from build123d import *

# Parameters (mm, degrees)
F0_W          = 20
F0_H          = 40
F0_R          = 1.75
F1_DEPTH      = 14
F2_W          = 20
F2_H          = 8.7217967697
F2_H_2        = 9.1349255253
F3_DEPTH      = 10
F4_R          = 6
F5_DEPTH      = 14
F5_DEPTH_BACK = 20


with BuildPart() as f1:
    # F0 (on Top) → F1 (new body)
    with BuildSketch(Plane.XY):
        Rectangle(F0_W, F0_H)
        with Locations((0, -15)):
            Circle(F0_R, mode=Mode.SUBTRACT)
        with Locations((0, 15)):
            Circle(F0_R, mode=Mode.SUBTRACT)
    extrude(amount=F1_DEPTH)

    # F2 (on face) → F3 (cut)
    with BuildSketch(Plane.XY.offset(14)):
        Polygon((-6.0882685902, -5.1451905284), (-3.75, -6.4951905284), (-1.3077413577, -7.8650744747), (6.4248711306, 5.5282032303), (1.6617314098, 8.2782032303), align=None)
        with Locations((0, 15.6391016151)):
            Rectangle(F2_W, F2_H)
        with Locations((0, -15.4325372373)):
            Rectangle(F2_W, F2_H_2)
    extrude(amount=-F3_DEPTH, mode=Mode.SUBTRACT)

    # F4 (on face) → F5 (cut, two sides)
    with BuildSketch(Plane(origin=(-2.3382685902, 1.35, 0), x_dir=(0.5, 0.8660254038, 0), z_dir=(0.8660254038, -0.5, 0))) as f5_sk:
        with Locations((0.25, 12.454691343)):
            Circle(F4_R)
    extrude(amount=-F5_DEPTH, mode=Mode.SUBTRACT)
    extrude(f5_sk.sketch, amount=F5_DEPTH_BACK, mode=Mode.SUBTRACT)


solid = f1.part
Geometry: final body of the model. Coordinates: model frame, mm. A direction names the side the tool comes from. Round coordinates to 2 decimals unless told otherwise and drop trailing zeros. Loops run counter-clockwise (first coordinate to the right, second up) from the corner with the lowest first, then second, coordinate; pieces in that order, holes last. Notation, with made-up numbers: (50, 11.25) - (66, 11.25) arc R28 cw to (66, 40.25) - close; hole circle Ø7 at (20, 51.5). An arc over 180 degrees is marked (long way). Write each question's results on one line, items separated by ' | '. Start each with the question number.
1) Cut plane C-C on z = 11. Return loops of the section in (x, y), then the cut area to 3 significant figures.
2) Cut plane B-B on y = 15. Return loops of the section in (x, z).
3) Cut plane D-D on z = 2.25. Return loops of the section in (x, y), then the cut area to 3 significant figures.
4) Cut plane A-A on z = 4.5. Return loops of the section in (x, y), then the cut area to 3 significant figures.
5) Mould query, pull axis Y, two halves, no side actions, for faces 4 (the face through (0, 20, 2)), 5 (the face through (-10, 0, 5)), 6 (the face through (2.504, -1.262, 5.737)), 7 (the face through (0, -10.865, 9)). Classes: released by +Y, released by -Y, zero draft, split by the parting line, or undercut.
6) Line query: probe 1 along Y at (x, z) = (0, 0.9); probe 2 along X at (y, z) = (15, 2); probe 3 along Z at (x, y) = (1, 4). Output: solid intervals per line, ascending. Write a range as [from, to].
7) Access query for faces 1 (the face through (0, -17, 4)), 2 (the face through (0, 18, 4)), 3 (the face through (0, 0, 4)). Directions: +Z, -Z, +X, -X, +Y, -Y. A direction counts if a zero-diameter tool reaches every point of the face in a straight line with its end or side. Return the directions, or none.
8) First-contact query: P1, Ø3, axis at x = 0, y = 15, coming from the -Z side; P2, Ø4, axis at x = 7, y = -7.5, coming from the +Z side; P3, Ø5, axis at x = 6.5, y = -6, coming from the -Z side; P4, Ø1, axis at y = 6.5, z = 12.5, coming from the -X side. Flat tips, straight axial feed; report the tip coordinate or a pass-through.
Verdict:
1) outline: (-10, -10.87) - (7.68, -10.87) - (-0.36, -6.22) - (-1.31, -7.87) - (-3.75, -6.5) - (-6.09, -5.15) - (-5.12, -3.47) - (-10, -0.66) - close; (-7.39, 11.28) - (0.7, 6.61) - (1.66, 8.28) - (6.42, 5.53) - (5.46, 3.86) - (10, 1.24) - (10, 11.28) - close | area: 156 mm2
2) outline: (-10, 0) - (-1.75, 0) - (-1.75, 4) - (-10, 4) - close; (1.75, 0) - (10, 0) - (10, 4) - (1.75, 4) - close
3) outline: (-10, -20) - (10, -20) - (10, 20) - (-10, 20) - close; hole circle Ø3.5 at (0, -15); hole circle Ø3.5 at (0, 15) | area: 781 mm2
4) outline: (-10, -10.87) - (10, -10.87) - (10, 11.28) - (-10, 11.28) - close; hole (-6.09, -5.15) - (-3.75, -6.5) - (-1.31, -7.87) - (6.42, 5.53) - (1.66, 8.28) - close | area: 358 mm2
5) face 4: released by +Y | face 5: zero draft | face 6: undercut | face 7: released by -Y
6) probe 1: y = [-20, -16.75], [-13.25, 13.25], [16.75, 20] | probe 2: x = [-10, -1.75], [1.75, 10] | probe 3: z = [0, 4]
7) face 1: +Z, +X, -X, -Y | face 2: +Z, +X, -X, +Y | face 3: +Z
8) P1: passes through | P2: stops at z = 9.54 | P3: stops at z = 0 | P4: stops at x = 0.38
